Geometry check sheet. Reference: the model listing, model coordinates, mm. A direction names the side the tool comes from. Coordinates: 2 decimals unless noted, no trailing zeros. Loops run counter-clockwise (first coordinate to the right, second up) from the corner with the lowest first, then second, coordinate; pieces in that order, holes last. Notation, with made-up numbers: (-23.75, 77) - (1.25, 77) arc R20 cw to (1.25, 97) - close; hole circle Ø7 at (20, 44.5). An arc over 180 degrees is marked (long way). One line per item, written item: value.
from build123d import *

# Parameters (mm, degrees)
F0_W     = 65.05388394
F0_H     = 41.2077661604
F1_DEPTH = 25.4
F2_W     = 65.05388394
F2_H     = 41.2077661604
F3_DEPTH = 25.4
F5_DEPTH = 4.572


with BuildPart() as f1:
    # F0 (on Front) → F1 (new body)
    with BuildSketch(Plane.XZ):
        with Locations((0.313764438, -2.9284702614)):
            Rectangle(F0_W, F0_H)
    extrude(amount=F1_DEPTH)

    # F2 (on face) → F3 (join)
    with BuildSketch(Plane.XZ.offset(25.4)):
        with Locations((0.313764438, -2.9284702614)):
            Rectangle(F2_W, F2_H)
        Polygon((-23.4277658165, -9.0991770849), (-23.4277658165, 2.8238825034), (0, -3.2422353979), align=None, mode=Mode.SUBTRACT)
        Polygon((20.9176484495, -9.0991770849), (0, -3.2422353979), (20.9176484495, 2.8238825034), align=None, mode=Mode.SUBTRACT)
        Polygon((0, -3.2422353979), (-23.4277658165, 2.8238825034), (-23.4277658165, -9.0991770849), align=None)
        Polygon((20.9176484495, 2.8238825034), (0, -3.2422353979), (20.9176484495, -9.0991770849), align=None)
    extrude(amount=F3_DEPTH)

    # F4 (on face) → F5 (join)
    with BuildSketch(Plane.XY.offset(17.6754128188)):
        Polygon((0, -25.8332956582), (-22.8002350777, -12.4460002407), (-22.8002350777, -36.292117089), (0, -28.3434130251), (25.5195293576, -36.292117089), (25.5195293576, -12.4460002407), align=None)
    extrude(amount=F5_DEPTH)


solid = f1.part
(1) Release check for a two-part mould opening along X. For faces 4 (the face through (1, -27, 22.247)), 5 (the face through (12.58, -32.26, 19.93)), 6 (the face through (-22.8, -24, 20)), 7 (the face through (25.52, -25, 20)) record: pulls with the +X half, pulls with the -X half, needs draft (parallel to the pull), parting line crosses it, or undercut.
Reply:
face 4: needs draft
face 5: undercut
face 6: pulls with the -X half
face 7: pulls with the +X half
(2) Go/stop test with flat-tipped pins: pin 1 Ø2.5 at (y, z) = (-27, 19.5) entering from -X; pin 2 Ø10 at (x, y) = (-1, -40) entering from +Z; pin 3 Ø2.5 at (y, z) = (-27.5, 20.5) entering from +X. Record where each tip stops, or that it passes through.
Reply:
pin 1: x = -22.8
pin 2: z = 17.68
pin 3: x = 25.52
(3) Cross-section at B-B on y = -8. Record the cut outline in (x, z).
Reply:
outline: (-32.21, -23.53) - (32.84, -23.53) - (32.84, 17.68) - (-32.21, 17.68) - close
(4) Access from +Z, -Z, +X, -X, +Y, -Y to the whole of each face (thin tool, end or side, straight path). Record for faces 1 (the face through (12.938, -19.046, 19.929)), 2 (the face through (-32.213, -25, -3)), 3 (the face through (-11.56, -32.373, 19.929)).
Reply:
face 1: +Z, +Y
face 2: +Z, -Z, -X, +Y, -Y
face 3: +Z, -Y
(5) Cross-section at A-A on x = 2.5. Record the cut outline in (y, z).
Reply:
outline: (-50.8, -23.53) - (0, -23.53) - (0, 17.68) - (-24.52, 17.68) - (-24.52, 22.25) - (-29.12, 22.25) - (-29.12, 17.68) - (-50.8, 17.68) - close
(6) Cross-section at C-C on x = 20. Record the cut outline in (y, z), and give its area (3 significant figures).
Reply:
outline: (-50.8, -23.53) - (0, -23.53) - (0, 17.68) - (-15.34, 17.68) - (-15.34, 22.25) - (-34.57, 22.25) - (-34.57, 17.68) - (-50.8, 17.68) - close
area: 2,180 mm2
(7) Material ranges on probe 1 along Z at (x, y) = (-26, -20.5); probe 2 along Y at (x, z) = (-18, 19), recorded low to high. Write a range as from..to.
Reply:
probe 1: -23.53..17.68
probe 2: -34.62..-15.26
